from build123d import *

# Parameters (mm, degrees)
F1_DEPTH = 1.016
F3_D     = 4.064
F4_R     = 1.778
F5_DEPTH = 2.032


with BuildPart() as f1:
    # F0 (on Top) → F1 (new body)
    with BuildSketch(Plane.XY):
        with BuildLine():
            ThreePointArc((-3.81, -3.81), (-1.115923, -2.694077), (0, 0))
            ThreePointArc((0, 0), (-1.115923, 2.694077), (-3.81, 3.81))
            ThreePointArc((-3.81, 3.81), (-7.62, 0), (-3.81, -3.81))
        make_face()
        with BuildLine():
            ThreePointArc((3.81, 3.81), (1.115923, 2.694077), (0, 0))
            ThreePointArc((0, 0), (1.115923, -2.694077), (3.81, -3.81))
            ThreePointArc((3.81, -3.81), (6.504077, -2.694077), (7.62, 0))
            ThreePointArc((7.62, 0), (6.504077, 2.694077), (3.81, 3.81))
        make_face()
        with BuildLine():
            ThreePointArc((3.81, -3.81), (1.115923, -2.694077), (0, 0))
            ThreePointArc((0, 0), (-1.115923, -2.694077), (-3.81, -3.81))
            Line((-3.81, -3.81), (3.81, -3.81))
        make_face()
        with BuildLine():
            ThreePointArc((-3.81, 3.81), (-1.115923, 2.694077), (0, 0))
            ThreePointArc((0, 0), (1.115923, 2.694077), (3.81, 3.81))
            Line((3.81, 3.81), (-3.81, 3.81))
        make_face()
    extrude(amount=F1_DEPTH)

    # F3 (through all)
    with Locations(Plane.XY.offset(1.016)):
        with Locations((3.81, 0)):
            Hole(F3_D / 2)

    # F4 (on face) → F5 (join)
    with BuildSketch(Plane.XY.offset(1.016)):
        with Locations((-3.81, 0)):
            Circle(F4_R)
    extrude(amount=F5_DEPTH)


solid = f1.part
CAD build for the part. Positions are in the model's coordinates, mm. Round coordinates to 2 decimals unless told otherwise and drop trailing zeros. Loops run counter-clockwise (first coordinate to the right, second up) from the corner with the lowest first, then second, coordinate; pieces in that order, holes last.
(1) Cut at C-C (x = -4.75). Give the cut face in (y, z).
(2) Cut at D-D (z = 1.8). Give the cut face in (x, y).
(3) Drop flat-ended pins along their axis: pin 1 (4.5 mm diameter, centred on x = 3.81, y = 0, fed in from -Z); pin 2 (1 mm diameter, centred on y = -1, z = 1, fed in from -X). Give the stop position or say it passes through.
(4) Cut at B-B (y = 1). Give the cut face in (x, z), plus the area to 3 significant figures.
(5) Two-plate mould, pull along Y, no slides. Class faces 1 (the cylindrical face through (1.933, -0.778, 0.501)), 2 (the cylindrical face through (-2.168, -0.681, 2.018)), 3 (the flat face through (-4, 0, 3.048)): +Y half, -Y half, draft (parallel to the pull), parting line (faces both ways), or undercut.
(6) Cut at A-A (z = 0.6). Give the cut face in (x, y), plus the area to 3 significant figures.
(7) Wall check: line 1 along Z through (x, y) = (6.25, 0.5); line 2 along X through (y, z) = (1.25, 0.65); line 3 along X through (y, z) = (-1.75, 0.95). Give the ranges that are in metal, low to high.
Findings below:
1. outline: (-3.69, 0) - (3.69, 0) - (3.69, 1.02) - (1.51, 1.02) - (1.51, 3.05) - (-1.51, 3.05) - (-1.51, 1.02) - (-3.69, 1.02) - close
2. outline: circle Ø3.56 at (-3.81, 0)
3. pin 1: stops at z = 0
3. pin 2: stops at x = -7.59
4. outline: (-7.49, 0) - (2.04, 0) - (2.04, 1.02) - (-2.34, 1.02) - (-2.34, 3.05) - (-5.28, 3.05) - (-5.28, 1.02) - (-7.49, 1.02) - close; (5.58, 0) - (7.49, 0) - (7.49, 1.02) - (5.58, 1.02) - close
4. area: 17.6 mm2
5. face 1: undercut
5. face 2: parting line
5. face 3: draft
6. outline: (-3.81, -3.81) - (3.81, -3.81) arc R3.81 ccw to (7.62, 0) arc R3.81 ccw to (3.81, 3.81) - (-3.81, 3.81) arc R3.81 ccw to start; hole circle Ø4.06 at (3.81, 0)
6. area: 90.7 mm2
7. line 1: z = 0 to 1.02
7. line 2: x = -7.41 to 2.21, 5.41 to 7.41
7. line 3: x = -7.19 to 2.78, 4.84 to 7.19
